```python
from build123d import *

# Parameters (mm, degrees)
SKETCH1_R           = 34.925
SKETCH1_R_2         = 30.1625
BOSS_EXTRUDE1_DEPTH = 50.8
SKETCH2_R           = 50.8
SKETCH2_R_2         = 44.45
BOSS_EXTRUDE2_DEPTH = 50.8
SKETCH4_R           = 30.1625
SKETCH4_R_2         = 29.21
BOSS_EXTRUDE3_DEPTH = 15.0876
CUT_EXTRUDE1_REACH  = 89.988
SKETCH6_R           = 2.2225


with BuildPart() as part:
    # Sketch1 → Boss-Extrude1 (new body)
    with BuildSketch(Plane(origin=(0, 0, 0), x_dir=(1, 0, 0), z_dir=(0, 1, 0))):
        with Locations(Location((0, 0, 0), (0, 0, 270))):
            Circle(SKETCH1_R)
        with Locations(Location((0, 0, 0), (0, 0, 270))):
            Circle(SKETCH1_R_2, mode=Mode.SUBTRACT)
    extrude(amount=BOSS_EXTRUDE1_DEPTH)



with BuildPart() as body_2:
    # Sketch2 → Boss-Extrude2 (new body)
    with BuildSketch(Plane(origin=(0, 50.8, 0), x_dir=(1, 0, 0), z_dir=(0, 1, 0))):
        with Locations(Location((0, 0, 0), (0, 0, 270))):
            Circle(SKETCH2_R)
        with Locations(Location((0, 0, 0), (0, 0, 270))):
            Circle(SKETCH2_R_2, mode=Mode.SUBTRACT)
    extrude(amount=BOSS_EXTRUDE2_DEPTH)


with BuildPart() as part_1:
    add(part.part)

    add(body_2.part)  # Revolve1 merges body 2
    # Sketch3 → Revolve1 (revolve)
    with BuildSketch(Plane.XY, mode=Mode.PRIVATE) as revolve1_sk:
        Polygon((50.8, 50.8), (34.925, 34.925), (34.925, 50.8), align=None)
    revolve(revolve1_sk.sketch.rotate(Axis((0, 101.6, 0), (0, -1, 0)), 90), axis=Axis((0, 101.6, 0), (0, -1, 0)))

    # Sketch4 → Boss-Extrude3 (add)
    with BuildSketch(Plane(origin=(0, 50.8, 0), x_dir=(1, 0, 0), z_dir=(0, 1, 0))):
        with Locations(Location((0, 0, 0), (0, 0, 270))):
            Circle(SKETCH4_R)
        with Locations(Location((0, 0, 0), (0, 0, 270))):
            Circle(SKETCH4_R_2, mode=Mode.SUBTRACT)
    extrude(amount=-BOSS_EXTRUDE3_DEPTH)

    # Sketch5 → Cut-Revolve1 (revolve, cut)
    with BuildSketch(Plane(origin=(0, 0, 0), x_dir=(0, 0, -1), z_dir=(1, 0, 0))):
        Polygon((-44.45, 50.8), (-29.21, 36.195), (-29.21, 50.8), align=None)
    revolve(axis=Axis((0, 101.6, 0), (0, -1, 0)), mode=Mode.SUBTRACT)

    # Cut-Extrude1: up to this cone (the profile starts inside it)
    cut_extrude1_end = Plane(origin=(0, 50.8, 0), z_dir=(0, 1, 0)).offset(-50.799999) * Cone(1e-06, 192.088, 192.087999, align=(Align.CENTER, Align.CENTER, Align.MIN), mode=Mode.PRIVATE)
    # Sketch6 → Cut-Extrude1 (cut, up to the surface)
    with BuildSketch(Plane(origin=(0, 50.8, 0), x_dir=(-1, 0, 0), z_dir=(0, -1, 0)), mode=Mode.PRIVATE) as cut_extrude1_sk1:
        with Locations(Location((36.068, 0, 0), (0, 0, 237.524024199))):
            Circle(SKETCH6_R)
    cut_extrude1_tool1 = extrude(cut_extrude1_sk1.sketch, amount=CUT_EXTRUDE1_REACH, mode=Mode.PRIVATE) & cut_extrude1_end
    add(cut_extrude1_tool1.solids().sort_by_distance((-36.068, 50.8, 0))[0], mode=Mode.SUBTRACT)


solid = part_1.part
```
Build history of the part. All positions in model axes, mm. A direction names the side the tool comes from. Give positions to 0.01 mm unless a question says otherwise; leave off trailing zeros. Loops run counter-clockwise (first coordinate to the right, second up) from the corner with the lowest first, then second, coordinate; pieces in that order, holes last.
Item 1: Which spindle directions (+Z, -Z, +X, -X, +Y, -Y) get a long thin tool onto all of the face, cutting with end or side? Do faces 4 (the face through (-30.911, 75.844, -40.313)), 5 (the face through (16, 35.712, -25)), 6 (the face through (37.48, 75.84, 23.9)). Say none if no direction does.
Answers follow:
face 4: +Y, -Y
face 5: -Y
face 6: +Y
Item 2: Drill centre lines: line 1 (X direction, y = 76, z = 0); line 2 (X direction, y = 15.5, z = 0) (1 decimal); line 3 (Z direction, x = -7, y = 79). Where is each one in solid material? Low to high.
Answers follow:
line 1: x = -50.8 to -44.45, 44.45 to 50.8
line 2: x = -34.9 to -30.2, 30.2 to 34.9
line 3: z = -50.32 to -43.9, 43.9 to 50.32
Item 3: Slice it at D-D, the plane y = 80. List the corners of the cut face in (x, z), and give its area (3 significant figures).
Answers follow:
outline: circle Ø101.6 at (0, 0); hole circle Ø88.9 at (0, 0)
area: 1,900 mm2
Item 4: Pull direction X, two halves, no side cores. Call faces 1 (the face through (-10, 0, -29)), 2 (the face through (-34.094, 17.218, -7.571)), 3 (the face through (1.326, 17.606, -30.133)): released by +X, released by -X, zero draft, split by the parting line, or undercut.
Answers follow:
face 1: zero draft
face 2: split by the parting line
face 3: undercut
Item 5: Flat gauge pins, fed straight in: pin 1 (12 mm diameter, centred on y = 89, z = -30.5, fed in from +X); pin 2 (2 mm diameter, centred on y = 63, z = 5, fed in from +X); pin 3 (6 mm diameter, centred on y = 64, z = 17.5, fed in from +X). Where does each tip first touch, or does it go through?
Answers follow:
pin 1: stops at x = 44.5
pin 2: stops at x = 50.64
pin 3: stops at x = 48.69
Item 6: Slice it at B-B, the plane z = 0. Give the number of separate pieces and of enclosed holes in the cut face, and give its area (3 significant figures).
Answers follow:
separate pieces: 3
enclosed holes: 0
area: 1,160 mm2
